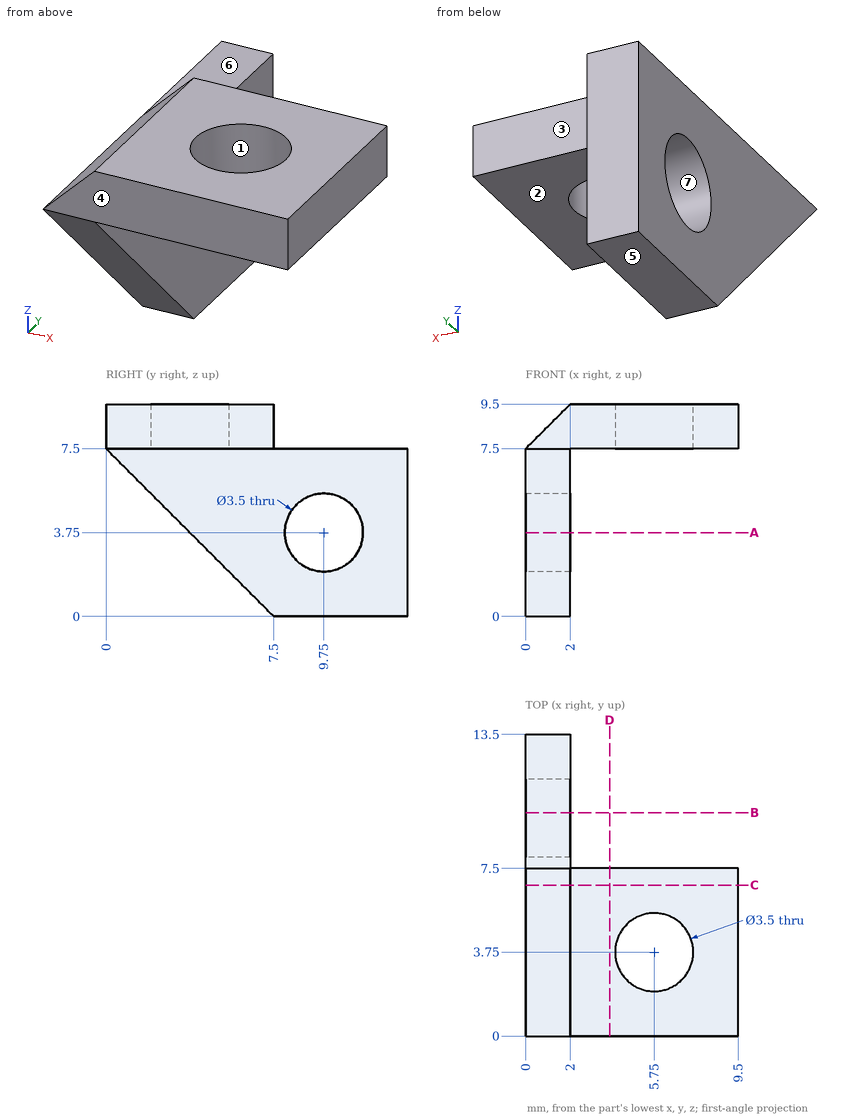
The figure shows three views and two pictorial views of one solid part (mm, origin at its lowest corner). Answer the questions. A direction names the side the tool comes from. Round coordinates to 2 decimals unless told otherwise and drop trailing zeros. Order: outer loops, then holes, each group sorted by start corner. A loop starts at its lowest first (then second) coordinate and runs counter-clockwise, first axis right, second up.
Q1. A cutting plane is placed at C-C, the plane y = 6.75. Determine the outline of the cut face in (x, z).
Solution:
outline: (0, 0.75) - (2, 0.75) - (2, 7.5) - (9.5, 7.5) - (9.5, 9.5) - (2, 9.5) - (0, 7.5) - close
Q2. The mould has two halves that part along Z. Classify the marked faces 4, 5, 6 and 7: pulls with the +Z half, pulls with the -Z half, needs draft (parallel to the pull), parting line crosses it, or undercut.
Solution:
face 4: needs draft
face 5: pulls with the -Z half
face 6: pulls with the +Z half
face 7: undercut
Q3. A tool of negligible diameter and unlimited length cuts with its end or side. For the marked faces 1, 2 and 3, from which of +Z, -Z, +X, -X, +Y, -Y can it reach the whole face along a straight path? Write none if from no direction.
Solution:
face 1: +Z, -Z
face 2: -Z, +X, +Y, -Y
face 3: +Z, +X, -X, +Y
Q4. A cutting plane is placed at B-B, the plane y = 10. Determine the outline of the cut face in (x, z).
Solution:
outline: (0, 0) - (2, 0) - (2, 2.02) - (0, 2.02) - close; (0, 5.48) - (2, 5.48) - (2, 7.5) - (0, 7.5) - close
Q5. A cutting plane is placed at D-D, the plane x = 3.75. Determine the outline of the cut face in (y, z), then the cut area to 3 significant figures.
Solution:
outline: (0, 7.5) - (7.5, 7.5) - (7.5, 9.5) - (0, 9.5) - close
area: 15.0 mm2
Q6. Find the intervals of material crossed by line 1 along Z through (x, y) = (1.6, 9.75); line 2 along Z through (x, y) = (1.75, 9.25); line 3 along Z through (x, y) = (3, 1), in increasing order.
Solution:
line 1: z = 0 to 2, 5.5 to 7.5
line 2: z = 0 to 2.07, 5.43 to 7.5
line 3: z = 7.5 to 9.5
Q7. A cutting plane is placed at A-A, the plane z = 3.75. Determine the outline of the cut face in (x, y), then the cut area to 3 significant figures.
Solution:
outline: (0, 3.75) - (2, 3.75) - (2, 8) - (0, 8) - close; (0, 11.5) - (2, 11.5) - (2, 13.5) - (0, 13.5) - close
area: 12.5 mm2
Q8. Given pin 1 Ø0.6 at (x, y) = (1, 9.5) entering from +Z; pin 2 Ø2 at (x, y) = (5, 4.5) entering from -Z; pin 3 Ø2 at (y, z) = (8, 2) entering from +X, each flat-ended and moving along its own axis, determine where each tip first touches the part or whether it passes through.
Solution:
pin 1: stops at z = 7.5
pin 2: stops at z = 7.5
pin 3: stops at x = 2
